Here's how the part is built. I have some questions about the finished solid (model axes, mm). A direction names the side the tool comes from. Round coordinates to 2 decimals unless told otherwise and drop trailing zeros. Loops run counter-clockwise (first coordinate to the right, second up) from the corner with the lowest first, then second, coordinate; pieces in that order, holes last. Notation, with made-up numbers: (74, 16) -> (87, 16) arc R14 cw to (87, 26) -> close; hole circle Ø8 at (-1, -4.5). An arc over 180 degrees is marked (long way). Use one line per item in the form item = value. Start each with the question number.
Item 1: If we section it at D-D (x = -46.5): Write out the boundary of the cut face in (y, z), then the cut area to 3 significant figures.
Item 2: I'm going to push flat-ended pins straight in: pin 1 Ø1 at (x, z) = (-35.5, -36.5) entering from +Y; pin 2 Ø3 at (y, z) = (-23.5, -0.5) entering from -X; pin 3 Ø1 at (x, y) = (-45.5, -24) entering from -Z. Where does each tip first touch, or does it pass through?
Item 3: If we section it at C-C (y = -24.25): Write out the boundary of the cut face in (x, z), then the cut area to 3 significant figures.
Item 4: For faces 4 (the face through (-34, -20, -34)), 5 (the face through (-49, -22, -17.901)), 6 (the face through (-45, -21, -35.901)), 7 (the face through (-34, -21.936, -37)), which set-ups out of +Z, -Z, +X, -X, +Y, -Y let a thin tool reach every point of the face, with its end or its side?
Item 5: If we section it at A-A (y = -20.75): Write out the boundary of the cut face in (x, z), then the cut area to 3 significant figures.
Item 6: Thinking about a two-plate mould opening in X: for faces 1 (the face through (-41.142, -22, 6)), 2 (the face through (-27.712, -21.978, 31.027)), 3 (the face through (-34.166, -21.08, -15.803)), which applies, released by +X, released by -X, zero draft, split by the parting line, or undercut?
Item 7: If we section it at B-B (z = 23.5): Write out the boundary of the cut face in (x, y).
Item 8: If I drill on L1, parallel to X at y = -19.75, z = 8; L2, parallel to X at y = -22, z = 4.5; L3, parallel to Z at x = -45.5, y = -24.5, over which ranges is the centre line in solid material (lowest first)? Write a range as [from, to].
Autodesk Inventor part; units mm, degrees
ref_plane "YZ Plane" through (0, 0, 0) normal (1, 0, 0) x (0, 1, 0)
ref_plane "XZ Plane" through (0, 0, 0) normal (0, 1, 0) x (-1, 0, 0)
ref_plane "XY Plane" through (0, 0, 0) normal (0, 0, 1) x (1, 0, 0)
ref_plane "РабПлоскость1" through (-30.8415, -18.9359, 233.6055) normal (0, -1, 0) x (1, 0, 0)
sketch "Эскиз1" plane through (-30.8415, -18.9359, 233.6055) normal (0, -1, 0) x (1, 0, 0)
  line L0 (-13.3, -2.4998) -> (-13.3, -252.4998)
  line L1 (6.7, -2.4998) -> (6.7, -252.4998)
  line L2 (-13.3, -201.9768) -> (6.7, -201.9768)
  line L3 (6.7, -201.9768) -> (6.7, -265.9768)
  line L4 (0.7, -271.9768) -> (-7.3, -271.9768)
  line L5 (-13.3, -265.9768) -> (-13.3, -201.9768)
  line L6 (-6.6, -2.4998) -> (-6.6, -252.4998)
  line L7 (0, -2.4998) -> (0, -252.4998)
  circle A0 centre (-3.3, -240.4998) radius 1.25
  circle A1 centre (-3.3, -225.4998) radius 1.25
  line L8 (-6.2394, -252.4998) -> (-3.6, -252.4998)
  arc A2 (-13.3, -265.9768) -> (-7.3, -271.9768) centre (-7.3, -265.9768) ccw
  arc A3 (0.7, -271.9768) -> (6.7, -265.9768) centre (0.7, -265.9768) ccw
  circle A4 centre (-3.3, -260.4999) radius 3.3
  point P0 (30.8415, -233.6055)
  point P1 (-13.3, -271.9768)
  point P2 (-4.9197, -252.4998)
  dimension "d0" = 70
  dimension "d1" = 15
  dimension "d2" = 2.5
  dimension "d3" = 2.5
  dimension "d4" = 3.3
  dimension "d5" = 12
  dimension "d6" = 6
extrude "Выдавливание1" add sketch "Эскиз1" along normal blind 3
sketch "Эскиз2" plane through (-30.8415, -21.9359, 233.6055) normal (0, -1, 0) x (1, 0, 0)
  line L0 (-13.3, -201.9768) -> (-13.3, -265.9768)
  line L1 (-13.3, -248.5067) -> (-13.3, -271.9768)
  line L2 (-13.3, -271.9768) -> (6.7, -271.9768)
  line L3 (6.7, -271.9768) -> (6.7, -248.5067)
  line L4 (6.7, -265.9768) -> (6.7, -201.9768)
  line L5 (-13.3, -248.5067) -> (6.7, -248.5067)
  point P0 (30.8415, -233.6055)
  point P1 (0.7, -271.9768)
extrude "Выдавливание2" cut sketch "Эскиз2" against normal blind 3
sketch "Эскиз3" plane through (-30.8415, -21.9359, 233.6055) normal (0, -1, 0) x (1, 0, 0)
  line L0 (-13.3, -201.9768) -> (-13.3, -248.5067)
  line L1 (-13.3, -244.5067) -> (6.7, -244.5067)
  line L2 (6.7, -244.5067) -> (6.7, -271.5067)
  line L3 (6.7, -271.5067) -> (-13.3, -271.5067)
  line L4 (-13.3, -271.5067) -> (-13.3, -244.5067)
  line L5 (6.7, -248.5067) -> (6.7, -201.9768)
  line L6 (-13.3, -248.5067) -> (6.7, -248.5067)
  circle A0 centre (-3.3, -260.4998) radius 2.5
  circle A1 centre (-3.3, -260.4998) radius 2.25
  point P0 (30.8415, -233.6055)
  dimension "d11" = 27
  dimension "d12" = 4
  dimension "d22" = 4.5
extrude "Выдавливание3" add sketch "Эскиз3" along normal blind 3 contours L1 L2 L6 L0 | L6 L2 L3 L4 | A0
fillet "Сопряжение1" radius 3 3 edges at (-34.1415, -21.9359, -10.9012) (-34.1415, -21.9359, -14.9012) (-34.1415, -24.9359, -10.9012)
fillet "Сопряжение2" radius 3 4 edges at (-44.1415, -23.4359, -37.9012) (-24.1415, -23.4359, -37.9012) (-44.1415, -20.4359, 31.6287) (-24.1415, -20.4359, 31.6287)
sketch "Эскиз4" plane through (-30.8415, -21.9359, 233.6055) normal (0, -1, 0) x (1, 0, 0)
  arc A0 (3.7, -271.5067) -> (6.7, -268.5067) centre (3.7, -268.5067) ccw
  line L0 (3.7, -271.5067) -> (6.7, -271.5067)
  line L1 (6.7, -271.5067) -> (6.7, -201.9768)
  line L2 (6.7, -201.9768) -> (3.7, -201.9768)
  line L3 (3.7, -201.9768) -> (3.7, -271.5067)
  arc A1 (-13.3, -268.5067) -> (-10.3, -271.5067) centre (-10.3, -268.5067) ccw
  line L4 (-10.3, -271.5067) -> (-13.3, -271.5067)
  line L5 (-13.3, -271.5067) -> (-13.3, -201.9768)
  line L6 (-13.3, -201.9768) -> (-10.3, -201.9768)
  line L7 (-10.3, -201.9768) -> (-10.3, -271.5067)
  point P0 (30.8415, -233.6055)
  point P1 (-13.3, -268.5067)
  point P2 (6.7, -268.5067)
extrude "Выдавливание4" cut sketch "Эскиз4" along normal blind 10 and the other way blind 5 contours L3 L2 L1 A0 | L5 L6 L7 A1
fillet "Сопряжение3" radius 2 4 edges at (-41.1415, -23.4359, -37.9012) (-27.1415, -23.4359, -37.9012) (-27.1415, -20.4359, 31.6287) (-41.1415, -20.4359, 31.6287)
sketch "Эскиз5" plane through (-30.8415, -24.9359, 233.6055) normal (0, -1, 0) x (1, 0, 0)
  arc A0 (1.7, -271.5067) -> (3.7, -269.5067) centre (1.7, -269.5067) ccw
  line L0 (3.7, -269.5067) -> (3.7, -247.5067)
  line L1 (-10.3, -247.5067) -> (3.7, -247.5067)
  line L2 (-10.3, -247.5067) -> (-10.3, -269.5067)
  arc A1 (-10.3, -269.5067) -> (-8.3, -271.5067) centre (-8.3, -269.5067) ccw
  line L3 (-8.3, -271.5067) -> (1.7, -271.5067)
  circle A2 centre (-3.3, -260.4998) radius 2.25
  arc A3 (-8.3, -201.9768) -> (-10.3, -203.9768) centre (-8.3, -203.9768) ccw
  line L4 (-10.3, -203.9768) -> (-10.3, -242.3106)
  line L5 (3.7, -242.3106) -> (-10.3, -242.3106)
  line L6 (3.7, -242.3106) -> (3.7, -203.9768)
  arc A4 (3.7, -203.9768) -> (1.7, -201.9768) centre (1.7, -203.9768) ccw
  line L7 (1.7, -201.9768) -> (-8.3, -201.9768)
  circle A5 centre (-3.3, -225.4998) radius 1.25
  circle A6 centre (-3.3, -240.4998) radius 1.25
  line L8 (-10.3, -242.3106) -> (-10.3, -244.9086)
  line L9 (-10.3, -244.9086) -> (3.7, -244.9086)
  line L10 (3.7, -244.9086) -> (3.7, -242.3106)
  line L11 (3.7, -242.3106) -> (-10.3, -242.3106)
  line L12 (-10.3, -244.9086) -> (-10.3, -247.5067)
  line L13 (-10.3, -247.5067) -> (3.7, -247.5067)
  line L14 (3.7, -247.5067) -> (3.7, -244.9086)
  line L15 (-10.3, -244.9086) -> (3.7, -244.9086)
  point P0 (30.8415, -233.6055)
sketch "Эскиз6" plane through (-30.8415, -24.9359, 233.6055) normal (0, -1, 0) x (1, 0, 0)
  line L0 (-10.3, -269.5067) -> (-26.3, -269.5067)
  circle A0 centre (-23.3, -260.9834) radius 2.25
  line L1 (3.7, -269.5067) -> (3.7, -247.5067)
  line L2 (3.7, -244.9086) -> (3.7, -247.5067)
  line L3 (3.7, -244.9086) -> (3.7, -242.3106)
  line L4 (3.7, -242.3106) -> (3.7, -203.9768)
  arc A1 (3.7, -203.9768) -> (1.7, -201.9768) centre (1.7, -203.9768) ccw
  line L5 (1.7, -201.9768) -> (-8.3, -201.9768)
  arc A2 (-8.3, -201.9768) -> (-10.3, -203.9768) centre (-8.3, -203.9768) ccw
  line L6 (-10.3, -203.9768) -> (-10.3, -242.3106)
  line L7 (-10.3, -242.3106) -> (-10.3, -244.9086)
  line L8 (-28.3, -267.5067) -> (-28.3, -253.5067)
  line L9 (-26.3, -251.5067) -> (-10.3, -251.5067)
  line L10 (-10.3, -244.9086) -> (-10.3, -251.5067)
  circle A3 centre (-3.3, -240.4998) radius 1.25
  circle A4 centre (-3.3, -225.4998) radius 1.25
  arc A5 (-28.3, -267.5067) -> (-26.3, -269.5067) centre (-26.3, -267.5067) ccw
  arc A6 (-26.3, -251.5067) -> (-28.3, -253.5067) centre (-26.3, -253.5067) ccw
  line L11 (3.7, -251.5067) -> (3.7, -269.5067)
  line L12 (-10.3, -269.5067) -> (3.7, -269.5067)
  line L13 (-5.5991, -265.3019) -> (-5.5991, -250.3019)
  line L14 (-0.9846, -265.3019) -> (-0.9846, -250.3019)
  arc A7 (-5.5991, -265.3019) -> (-0.9846, -265.3019) centre (-3.2919, -265.3019) ccw
  arc A8 (-0.9846, -250.3019) -> (-5.5991, -250.3019) centre (-3.2919, -250.3019) ccw
  circle A9 centre (-3.3, -260.4998) radius 2.25
  point P0 (30.8415, -233.6055)
  point P1 (-28.3, -269.5067)
  point P2 (-18.3, -251.5067)
  dimension "d23" = 20
  dimension "d24" = 18
  dimension "d25" = 18
  dimension "d26" = 2
  dimension "d27" = 15
extrude "Выдавливание5" add sketch "Эскиз6" against normal blind 6 contours L0 A5 L8 A6 L9 L10 L7 L6 A2 L5 A1 L4 L3 L2 L1 L12
properties part number "крепление шкива боковое"
Values found:
q1.outline = (-24.94, -35.9) -> (-18.94, -35.9) -> (-18.94, -17.9) -> (-24.94, -17.9) -> close
q1.area = 108 mm2
q2.pin_1 = -21.94
q2.pin_2 = -41.14
q2.pin_3 = -35.9
q3.outline = (-59.14, -33.9) arc R2 ccw to (-57.14, -35.9) -> (-41.14, -35.9) arc R2 ccw to (-39.14, -37.9) -> (-29.14, -37.9) arc R2 ccw to (-27.14, -35.9) -> (-27.14, 29.63) arc R2 ccw to (-29.14, 31.63) -> (-39.14, 31.63) arc R2 ccw to (-41.14, 29.63) -> (-41.14, -17.9) -> (-57.14, -17.9) arc R2 ccw to (-59.14, -19.9) -> close; hole circle Ø4.5 at (-54.14, -27.38); hole circle Ø4.5 at (-34.14, -26.89); hole circle Ø2.5 at (-34.14, -6.89); hole circle Ø2.5 at (-34.14, 8.11)
q3.area = 1,250 mm2
q4.face_4 = +Y
q4.face_5 = +Z, -X, +Y, -Y
q4.face_6 = -Z, -X, +Y
q4.face_7 = -Z, +X, -X, +Y
q5.outline = (-59.14, -33.9) arc R2 ccw to (-57.14, -35.9) -> (-27.14, -35.9) -> (-27.14, 29.63) arc R2 ccw to (-29.14, 31.63) -> (-39.14, 31.63) arc R2 ccw to (-41.14, 29.63) -> (-41.14, -17.9) -> (-57.14, -17.9) arc R2 ccw to (-59.14, -19.9) -> close; hole circle Ø4.5 at (-54.14, -27.38); hole (-36.44, -31.7) arc R2.31 ccw to (-31.83, -31.7) -> (-31.83, -16.7) arc R2.31 ccw to (-32.15, -15.51) -> (-36.11, -15.51) arc R2.31 ccw to (-36.44, -16.7) -> close; hole circle Ø2.5 at (-34.14, -6.89); hole circle Ø2.5 at (-34.14, 8.11)
q5.area = 1,160 mm2
q6.face_1 = released by -X
q6.face_2 = released by +X
q6.face_3 = undercut
q7.outline = (-41.14, -24.94) -> (-27.14, -24.94) -> (-27.14, -18.94) -> (-41.14, -18.94) -> close
q8.L1 = [-41.14, -35.39], [-32.9, -27.14]
q8.L2 = [-41.14, -27.14]
q8.L3 = [-35.9, -17.9]
